Part model, mm, in its own coordinate system. Round coordinates to 2 decimals unless told otherwise and drop trailing zeros. Order: outer loops, then holes, each group sorted by start corner. A loop starts at its lowest first (then second) coordinate and runs counter-clockwise, first axis right, second up. Notation, with made-up numbers: M 83.5,44 L 120.5,44 A30 cw 120.5,79 Z; hole C -4.5,75.25 d5. An arc over 180 degrees is marked long. Write each question's results on one line, items separated by ' | '. Start each with the question number.
1. Band-saw the part on B-B, the plane x = -23. List the corners of the cut face in (y, z), then the cut area to 3 significant figures.
2. Band-saw the part on C-C, the plane z = 2.15. Give the number of separate pieces and of enclosed holes in the cut face, then the cut area to 3 significant figures.
3. Probe L1, parallel to X at y = -51, z = 0.85; L2, parallel to Y at x = 29, z = 1.2; L3, parallel to Y at x = -69.85, z = 1.05. List the from-to ranges inside material, lowest first. Write a range as [from, to].
4. Drop flat-ended pins along their axis: pin 1 Ø4 at (x, y) = (-28.5, -112.5) entering from -Z; pin 2 Ø1.5 at (x, z) = (10, 2.5) entering from +Y. Give the stop position or say it passes through.
5. Two-plate mould, pull along X, no slides. Class faces 1 (the face through (24.35, 12.098, 1.503)), 2 (the face through (-20, -11, 0)): +X half, -X half, draft (parallel to the pull), parting line (faces both ways), or undercut.
6. Band-saw the part on A-A, the plane x = -69.85. List the corners of the cut face in (y, z).
```python
from build123d import *

# Parameters (mm, degrees)
SKETCH1_W           = 165.1
SKETCH1_H           = 292.1
BOSS_EXTRUDE1_DEPTH = 3.048
SKETCH2_R           = 10.7315
SKETCH2_R_2         = 2.0193
SKETCH2_W           = 16.173788568
SKETCH2_H           = 32.6898
SKETCH2_W_2         = 76.2
SKETCH2_H_2         = 76.2
CUT_EXTRUDE1_DEPTH  = 168.792715289
CUT_EXTRUDE2_DEPTH  = 168.792715289
SKETCH5_R           = 2.54
CUT_EXTRUDE3_DEPTH  = 168.792715289
SKETCH6_W           = 165.1
SKETCH6_H           = 5.08
CUT_EXTRUDE4_DEPTH  = 168.792715289
CUT_EXTRUDE5_REACH  = 165.39
SKETCH7_R           = 5.08


with BuildPart() as part:
    # Sketch1 → Boss-Extrude1 (new body)
    with BuildSketch(Plane.XY):
        Rectangle(SKETCH1_W, SKETCH1_H)
    extrude(amount=BOSS_EXTRUDE1_DEPTH)

    # Sketch2 → Cut-Extrude1 (cut, through all)
    with BuildSketch(Plane.XY):
        with Locations((0, 92.71)):
            Circle(SKETCH2_R)
        with Locations(Location((0, 38.1, 0), (0, 0, 180))):
            Circle(SKETCH2_R_2)
        with Locations(Location((0, 30.1, 0), (0, 0, 180))):
            Circle(SKETCH2_R_2)
        with Locations(Location((0, 22.1, 0), (0, 0, 180))):
            Circle(SKETCH2_R_2)
        with Locations(Location((0, 14.1, 0), (0, 0, 180))):
            Circle(SKETCH2_R_2)
        with Locations(Location((0, 6.1, 0), (0, 0, 180))):
            Circle(SKETCH2_R_2)
        with Locations(Location((0, -1.9, 0), (0, 0, 180))):
            Circle(SKETCH2_R_2)
        with Locations(Location((0, -9.9, 0), (0, 0, 180))):
            Circle(SKETCH2_R_2)
        with Locations(Location((0, -17.9, 0), (0, 0, 180))):
            Circle(SKETCH2_R_2)
        with Locations(Location((-8, 38.1, 0), (0, 0, 180))):
            Circle(SKETCH2_R_2)
        with Locations(Location((-16, 38.1, 0), (0, 0, 180))):
            Circle(SKETCH2_R_2)
        with Locations(Location((-8, 30.1, 0), (0, 0, 180))):
            Circle(SKETCH2_R_2)
        with Locations(Location((-16, 30.1, 0), (0, 0, 180))):
            Circle(SKETCH2_R_2)
        with Locations(Location((-8, 22.1, 0), (0, 0, 180))):
            Circle(SKETCH2_R_2)
        with Locations(Location((-16, 22.1, 0), (0, 0, 180))):
            Circle(SKETCH2_R_2)
        with Locations(Location((-8, 14.1, 0), (0, 0, 180))):
            Circle(SKETCH2_R_2)
        with Locations(Location((-16, 14.1, 0), (0, 0, 180))):
            Circle(SKETCH2_R_2)
        with Locations(Location((-8, 6.1, 0), (0, 0, 180))):
            Circle(SKETCH2_R_2)
        with Locations(Location((-16, 6.1, 0), (0, 0, 180))):
            Circle(SKETCH2_R_2)
        with Locations(Location((-8, -1.9, 0), (0, 0, 180))):
            Circle(SKETCH2_R_2)
        with Locations(Location((-16, -1.9, 0), (0, 0, 180))):
            Circle(SKETCH2_R_2)
        with Locations(Location((-8, -9.9, 0), (0, 0, 180))):
            Circle(SKETCH2_R_2)
        with Locations(Location((-16, -9.9, 0), (0, 0, 180))):
            Circle(SKETCH2_R_2)
        with Locations(Location((-8, -17.9, 0), (0, 0, 180))):
            Circle(SKETCH2_R_2)
        with Locations(Location((-16, -17.9, 0), (0, 0, 180))):
            Circle(SKETCH2_R_2)
        with Locations(Location((24.086894284, 14.1, 0), (0, 0, 180))):
            Circle(SKETCH2_R_2)
        with Locations(Location((8.086894284, 14.1, 0), (0, 0, 180))):
            Circle(SKETCH2_R_2)
        with Locations(Location((8.086894284, -17.9, 0), (0, 0, 180))):
            Circle(SKETCH2_R_2)
        with Locations(Location((24.086894284, 6.1, 0), (0, 0, 180))):
            Circle(SKETCH2_R_2)
        with Locations(Location((16.086894284, 6.1, 0), (0, 0, 180))):
            Circle(SKETCH2_R_2)
        with Locations(Location((8.086894284, -1.9, 0), (0, 0, 180))):
            Circle(SKETCH2_R_2)
        with Locations(Location((8.086894284, 30.1, 0), (0, 0, 180))):
            Circle(SKETCH2_R_2)
        with Locations(Location((24.086894284, 22.1, 0), (0, 0, 180))):
            Circle(SKETCH2_R_2)
        with Locations(Location((24.086894284, -1.9, 0), (0, 0, 180))):
            Circle(SKETCH2_R_2)
        with Locations(Location((24.086894284, -9.9, 0), (0, 0, 180))):
            Circle(SKETCH2_R_2)
        with Locations(Location((8.086894284, 6.1, 0), (0, 0, 180))):
            Circle(SKETCH2_R_2)
        with Locations(Location((16.086894284, 22.1, 0), (0, 0, 180))):
            Circle(SKETCH2_R_2)
        with Locations(Location((8.086894284, 22.1, 0), (0, 0, 180))):
            Circle(SKETCH2_R_2)
        with Locations(Location((8.086894284, -9.9, 0), (0, 0, 180))):
            Circle(SKETCH2_R_2)
        with Locations(Location((24.086894284, -17.9, 0), (0, 0, 180))):
            Circle(SKETCH2_R_2)
        with Locations(Location((16.086894284, 14.1, 0), (0, 0, 180))):
            Circle(SKETCH2_R_2)
        with Locations(Location((16.086894284, -17.9, 0), (0, 0, 180))):
            Circle(SKETCH2_R_2)
        with Locations(Location((16.086894284, 30.1, 0), (0, 0, 180))):
            Circle(SKETCH2_R_2)
        with Locations(Location((24.086894284, 30.1, 0), (0, 0, 180))):
            Circle(SKETCH2_R_2)
        with Locations(Location((16.086894284, -9.9, 0), (0, 0, 180))):
            Circle(SKETCH2_R_2)
        with Locations(Location((16.086894284, -1.9, 0), (0, 0, 180))):
            Circle(SKETCH2_R_2)
        with Locations(Location((16.086894284, 38.1, 0), (0, 0, 180))):
            Circle(SKETCH2_R_2)
        with Locations(Location((8.086894284, 38.1, 0), (0, 0, 180))):
            Circle(SKETCH2_R_2)
        with Locations(Location((24.086894284, 38.1, 0), (0, 0, 180))):
            Circle(SKETCH2_R_2)
        with Locations((0, 92.71)):
            Rectangle(SKETCH2_W, SKETCH2_H)
        with Locations((0, -59.69)):
            Rectangle(SKETCH2_W_2, SKETCH2_H_2)
    extrude(amount=CUT_EXTRUDE1_DEPTH, mode=Mode.SUBTRACT)

    # Sketch4 → Cut-Extrude2 (cut, through all)
    with BuildSketch(Plane.XY):
        Polygon((-12.7, 57.310847547), (-12.7, 69.85), (-82.55, 69.85), (-82.55, 146.05), (82.55, 146.05), (82.55, 69.85), (12.7, 69.85), (12.7, 57.310847547), align=None)
    extrude(amount=CUT_EXTRUDE2_DEPTH, mode=Mode.SUBTRACT)

    # Sketch5 → Cut-Extrude3 (cut, through all)
    with BuildSketch(Plane(origin=(0, 0, 0), x_dir=(-1, 0, 0), z_dir=(0, 0, -1))):
        with Locations((-44.45, -106.299)):
            Circle(SKETCH5_R)
        with Locations((-69.85, -106.299)):
            Circle(SKETCH5_R)
        with Locations((69.85, -106.299)):
            Circle(SKETCH5_R)
        with Locations((44.45, -106.299)):
            Circle(SKETCH5_R)
    extrude(amount=-CUT_EXTRUDE3_DEPTH, mode=Mode.SUBTRACT)

    # Sketch6 → Cut-Extrude4 (cut, through all)
    with BuildSketch(Plane(origin=(0, 0, 0), x_dir=(-1, 0, 0), z_dir=(0, 0, -1))):
        with Locations((0, -143.51)):
            Rectangle(SKETCH6_W, SKETCH6_H)
    extrude(amount=-CUT_EXTRUDE4_DEPTH, mode=Mode.SUBTRACT)

    # Sketch7 → Cut-Extrude5 (cut, up to next)
    with BuildSketch(Plane.XY.offset(3.048), mode=Mode.PRIVATE) as cut_extrude5_sk1:
        with Locations((0, 57.310847547)):
            Circle(SKETCH7_R)
    cut_extrude5_tool1 = extrude(cut_extrude5_sk1.sketch, amount=-CUT_EXTRUDE5_REACH, mode=Mode.PRIVATE) & part.part
    add(cut_extrude5_tool1.solids().sort_by_distance((0, 57.310848, 3.048))[0], mode=Mode.SUBTRACT)


solid = part.part
```
Solution:
1) outline: M -140.97,0 L -97.79,0 L -97.79,3.05 L -140.97,3.05 Z; M -21.59,0 L 69.85,0 L 69.85,3.05 L -21.59,3.05 Z | area: 410 mm^2
2) separate pieces: 1 | enclosed holes: 53 | area: 27,900 mm^2
3) L1: [-82.55, -38.1], [38.1, 82.55] | L2: [-140.97, -97.79], [-21.59, 69.85] | L3: [-140.97, -108.84], [-103.76, 69.85]
4) pin 1: z = 0 | pin 2: y = 57.31
5) face 1: undercut | face 2: draft
6) outline: M -140.97,0 L -108.84,0 L -108.84,3.05 L -140.97,3.05 Z; M -103.76,0 L 69.85,0 L 69.85,3.05 L -103.76,3.05 Z
